Here's how the part is built. I have some questions about the finished solid (model axes, mm). Coordinates: 2 decimals unless noted, no trailing zeros. Write each loop counter-clockwise with the first axis right and the second up, starting at its lowest first coordinate (ties: lowest second). Pieces come first, ordered by that corner, then holes.
Item 1: I want a section at B-B (z = -10). Please give me the cut outline in (x, y).
Item 2: Please list where these lines run through material, in increasing order: line 1 (Z direction, x = 72, y = 2.25); line 2 (X direction, y = 4.25, z = -10); line 3 (Z direction, x = 24, y = 2.75).
Item 3: I want a section at A-A (y = 3.25). Please give me the cut outline in (x, z) (1 decimal).
Item 4: I'm going to push a flat-ended pin straight in: P1, Ø6, axis at x = 72, z = -10, coming from the +Y side. Where does the tip first touch, or does it pass through?
Item 5: I want a section at C-C (x = 72). Please give me the cut outline in (y, z).
Item 6: I want a section at D-D (x = -49). Please give me the cut outline in (y, z), and give its area (3 significant figures).
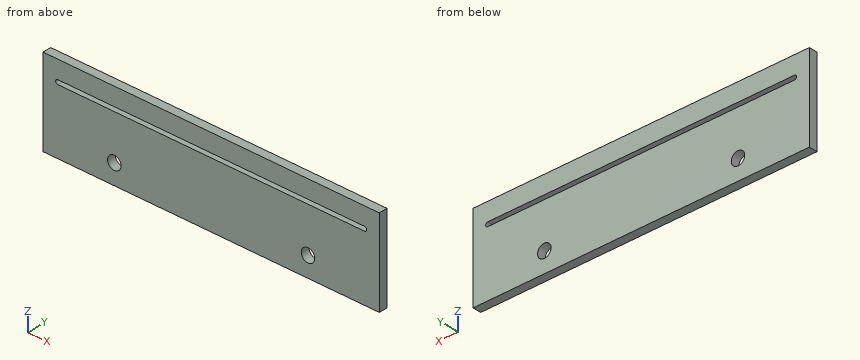
from build123d import *

# Parameters (mm, degrees)
SALIENTE_EXTRUIR1_DEPTH = 6.35
CROQUIS2_R              = 5
CORTAR_EXTRUIR3_DEPTH   = 7.35


with BuildPart() as part:
    # Croquis1 → Saliente-Extruir1 (new body)
    with BuildSketch(Plane(origin=(0, 0, 0), x_dir=(1, 0, 0), z_dir=(0, 1, 0))):
        Polygon((-125, -25), (-125, -40), (125, -40), (125, -25), (125, 25), (-125, 25), align=None)
    extrude(amount=SALIENTE_EXTRUIR1_DEPTH)

    # Croquis2 → Cortar-Extruir3 (cut, through all)
    with BuildSketch(Plane(origin=(0, 6.35, 0), x_dir=(1, 0, 0), z_dir=(0, 1, 0))):
        with Locations((-72, 10)):
            Circle(CROQUIS2_R)
        with Locations((72, 10)):
            Circle(CROQUIS2_R)
        with BuildLine():
            Line((114, -23.4125), (-114, -23.4125))
            ThreePointArc((-114, -23.4125), (-115.5875, -25), (-114, -26.5875))
            Line((-114, -26.5875), (114, -26.5875))
            ThreePointArc((114, -26.5875), (115.5875, -25), (114, -23.4125))
        make_face()
    extrude(amount=-CORTAR_EXTRUIR3_DEPTH, mode=Mode.SUBTRACT)


solid = part.part
Answer:
1. outline: (-125, 0) - (-77, 0) - (-77, 6.35) - (-125, 6.35) - close; (-67, 0) - (67, 0) - (67, 6.35) - (-67, 6.35) - close; (77, 0) - (125, 0) - (125, 6.35) - (77, 6.35) - close
2. line 1: z = -25 to -15, -5 to 23.41, 26.59 to 40
2. line 2: x = -125 to -77, -67 to 67, 77 to 125
2. line 3: z = -25 to 23.41, 26.59 to 40
3. outline: (-125, -25) - (125, -25) - (125, 40) - (-125, 40) - close; hole (-114, 23.4) - (114, 23.4) arc R1.6 ccw to (114, 26.6) - (-114, 26.6) arc R1.6 ccw to start; hole circle Ø10 at (-72, -10); hole circle Ø10 at (72, -10)
4. P1: passes through
5. outline: (0, -25) - (6.35, -25) - (6.35, -15) - (0, -15) - close; (0, -5) - (6.35, -5) - (6.35, 23.41) - (0, 23.41) - close; (0, 26.59) - (6.35, 26.59) - (6.35, 40) - (0, 40) - close
6. outline: (0, -25) - (6.35, -25) - (6.35, 23.41) - (0, 23.41) - close; (0, 26.59) - (6.35, 26.59) - (6.35, 40) - (0, 40) - close
6. area: 393 mm2
